Here's how the part is built. I have some questions about the finished solid (model axes, mm). A direction names the side the tool comes from. Round coordinates to 2 decimals unless told otherwise and drop trailing zeros. Write each loop counter-clockwise with the first axis right and the second up, starting at its lowest first coordinate (ties: lowest second). Pieces come first, ordered by that corner, then holes. Notation, with made-up numbers: (27.5, 47) -> (34.5, 47) arc R5 ccw to (34.5, 56) -> close; hole circle Ø11 at (-32, 56.25). An arc over 180 degrees is marked (long way). Put each result on its own line as item: value. Start each with the question number.
1) I want a section at D-D, the plane y = 83.5. List the corners of the cut face in (x, z) for me, then the cut area to 3 significant figures.
2) If I drill on line 1 along X through (y, z) = (-165, -38); line 2 along Z through (x, y) = (21, 261.5); line 3 along Y through (x, z) = (43, -68.5), over which ranges is the centre line in solid material (lowest first)? Write a range as [from, to].
3) Which directions (+Z, -Z, +X, -X, +Y, -Y) give clear straight access to the entire face, cutting with the end or side of a thin tool? Please do faces 1 (the flat face through (36.576, -4, -145)), 2 (the flat face through (46.101, 260, 1)), 3 (the flat face through (36.576, -4, 146)).
4) I want a section at A-A, the plane y = 255.5. List the corners of the cut face in (x, z) for me.
5) I want a section at C-C, the plane x = 10.5. List the corners of the cut face in (y, z) for me.
6) I want a section at B-B, the plane z = 31. List the corners of the cut face in (x, y) for me, then the cut area to 3 significant figures.
7) Will these pins go through, and if not, where does the flat tip stop? P1, Ø1.9, axis at x = 44, y = 261, coming from the -Z side; P2, Ø11, axis at x = 11, y = -36.5, coming from the +Z side; P3, Ø18.5, axis at y = -69.5, z = -149, coming from the -X side.
from build123d import *

# Parameters (mm, degrees)
F0_W     = 596.9
F0_H     = 254
F1_DEPTH = 36.576
F2_W     = 596.9
F2_H     = 327.152
F3_DEPTH = 3.175
F4_W     = 25.4
F4_H     = 152.4
F5_DEPTH = 6.35


with BuildPart() as f1:
    # F0 (on Right) → F1 (new body)
    with BuildSketch(Plane.YZ):
        Rectangle(F0_W, F0_H)
    extrude(amount=F1_DEPTH)

    # F2 (on face) → F3 (join)
    with BuildSketch(Plane.YZ.offset(36.576)):
        Rectangle(F2_W, F2_H)
    extrude(amount=F3_DEPTH)

    # F4 (on face) → F5 (join)
    with BuildSketch(Plane.YZ.offset(39.751)):
        with Locations((260.35, 0)):
            Rectangle(F4_W, F4_H)
    extrude(amount=F5_DEPTH)


solid = f1.part
Findings:
1. outline: (0, -127) -> (36.58, -127) -> (36.58, -163.58) -> (39.75, -163.58) -> (39.75, 163.58) -> (36.58, 163.58) -> (36.58, 127) -> (0, 127) -> close
1. area: 10,300 mm2
2. line 1: x = [0, 39.75]
2. line 2: z = [-127, 127]
2. line 3: y = [247.65, 273.05]
3. face 1: -Z, -X, +Y, -Y
3. face 2: +Z, -Z, +X, +Y, -Y
3. face 3: +Z, -X, +Y, -Y
4. outline: (0, -127) -> (36.58, -127) -> (36.58, -163.58) -> (39.75, -163.58) -> (39.75, -76.2) -> (46.1, -76.2) -> (46.1, 76.2) -> (39.75, 76.2) -> (39.75, 163.58) -> (36.58, 163.58) -> (36.58, 127) -> (0, 127) -> close
5. outline: (-298.45, -127) -> (298.45, -127) -> (298.45, 127) -> (-298.45, 127) -> close
6. outline: (0, -298.45) -> (39.75, -298.45) -> (39.75, 247.65) -> (46.1, 247.65) -> (46.1, 273.05) -> (39.75, 273.05) -> (39.75, 298.45) -> (0, 298.45) -> close
6. area: 23,900 mm2
7. P1: stops at z = -76.2
7. P2: stops at z = 127
7. P3: stops at x = 36.58
